Design review of the part built by this model. Coordinates are the model's own, in mm. Face numbers are marked on the shaded views. A direction names the side the tool comes from. Give positions to 0.01 mm unless a question says otherwise; leave off trailing zeros. Order: outer loops, then holes, each group sorted by start corner. A loop starts at its lowest first (then second) coordinate and runs counter-clockwise, first axis right, second up. Notation, with made-up numbers: (13, -31.5) -> (29, -31.5) arc R10 cw to (29, -16.5) -> close; hole circle Ø3 at (36.25, 79.5). An arc over 180 degrees is marked (long way). Return JSON: item names as keys, results as strings.
Solid Edge part; units mm, degrees
sketch "Sketch1" plane through (0, 0, 0) normal (0, 0, 1) x (1, 0, 0)
  circle A0 centre (0, 0) radius 22.5
extrude "Protrusion1" add sketch "Sketch1" against normal blind 5
sketch "Sketch2" plane through (0, 0, -5) normal (0, 0, -1) x (-1, 0, 0)
  circle A0 centre (-13.1417, 7.5798) radius 7
  circle A1 centre (0, 15.1709) radius 7
  circle A2 centre (13.1417, 7.5798) radius 7
extrude "ExtrudedProtrusion_2" add sketch "Sketch2" along normal blind 30
sketch "Sketch3" plane through (0, 0, 0) normal (0, 0, 1) x (1, 0, 0)
  circle A0 centre (13.1417, 7.5798) radius 6
  circle A1 centre (0, 15.1709) radius 6
  circle A2 centre (-13.1417, 7.5798) radius 6
extrude "ExtrudedCutout_2" cut sketch "Sketch3" against normal blind 33
fillet "Round_1" radius 1 3 edges at (-6, 15.1709, 0) (-19.1417, 7.5798, 0) (7.1417, 7.5798, 0)
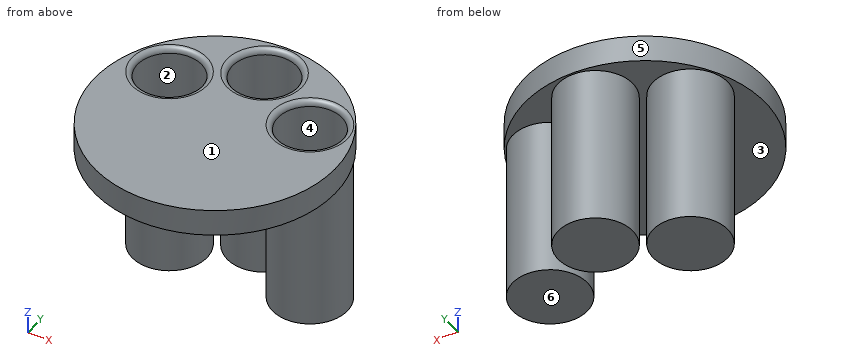
Item 1: Add section D-D (y = -2.5). Give the boundary of the cut face in (x, z), plus the area to 3 significant figures.
Result set:
{"outline": "(-22.36, -5) -> (22.36, -5) -> (22.36, 0) -> (-22.36, 0) -> close", "area": "224 mm^2"}
Item 2: Mouldability with a two-part tool opening along Y and no side actions: class the marked faces 4, 5 and 6 as released by +Y, released by -Y, zero draft, split by the parting line, or undercut.
Result set:
{"face 4": "undercut", "face 5": "split by the parting line", "face 6": "zero draft"}
Item 3: Add section A-A (z = -16.5). Give the boundary of the cut face in (x, y), plus the area to 3 significant figures.
Result set:
{"outline": "circle Ø14 at (-13.14, 7.58); circle Ø14 at (0, 15.17); circle Ø14 at (13.14, 7.58); hole circle Ø12 at (-13.14, 7.58); hole circle Ø12 at (0, 15.17); hole circle Ø12 at (13.14, 7.58)", "area": "123 mm^2"}
Item 4: Machinability: for the marked faces 1, 2 and 3, which of the approach directions +Z, -Z, +X, -X, +Y, -Y give a long, thin tool a straight path to every point of the face, cutting with its end or side? Answer none if there is none.
Result set:
{"face 1": "+Z, +X, -X, +Y, -Y", "face 2": "+Z", "face 3": "-Z"}
Item 5: For pin 1 (6 mm diameter, centred on x = 9.5, z = -18.5, fed in from -Y); pin 2 (9.5 mm diameter, centred on x = -13.14, y = 7.58, fed in from +Z); pin 3 (1 mm diameter, centred on x = -5.5, z = -28.5, fed in from -Y), all flat-tipped, find the tip position at first contact; note any pin that passes through.
Result set:
{"pin 1": "stops at y = 0.61", "pin 2": "stops at z = -33", "pin 3": "stops at y = 10.27"}
Item 6: Add section C-C (y = -16). Give the boundary of the cut face in (x, z), plus the area to 3 significant figures.
Result set:
{"outline": "(-15.82, -5) -> (15.82, -5) -> (15.82, 0) -> (-15.82, 0) -> close", "area": "158 mm^2"}
Item 7: Add section B-B (x = 0). Give the boundary of the cut face in (y, z), plus the area to 3 significant figures.
Result set:
{"outline": "(-22.5, -5) -> (8.17, -5) -> (8.17, -35) -> (22.17, -35) -> (22.17, -5) -> (22.5, -5) -> (22.5, 0) -> (22.17, 0) arc R1 ccw to (21.17, -1) -> (21.17, -33) -> (9.17, -33) -> (9.17, -1) arc R1 ccw to (8.17, 0) -> (-22.5, 0) -> close", "area": "249 mm^2"}
Item 8: Wall thickness on L1, parallel to X at y = 7.5, z = -7; L2, parallel to X at y = 6, z = -27.5; L3, parallel to X at y = 15, z = -25: over which ranges is each line inside the solid? List them lowest first. Write a range as [from, to].
Result set:
{"L1": "x = [-20.14, -19.14], [-7.14, -6.14], [6.14, 7.14], [19.14, 20.14]", "L2": "x = [-19.96, -18.93], [-7.35, -6.32], [6.32, 7.35], [18.93, 19.96]", "L3": "x = [-7, -6], [6, 7]"}
